Part model, mm, in its own coordinate system. A direction names the side the tool comes from. Coordinates: 2 decimals unless noted, no trailing zeros. Loops run counter-clockwise (first coordinate to the right, second up) from the corner with the lowest first, then second, coordinate; pieces in that order, holes last. Notation, with made-up numbers: M 22,-11.5 L 71,-11.5 A30 cw 71,25.5 Z; hole C 61,27 d5. An arc over 180 degrees is marked long. Use a Markdown table: item, result. Add a question column.
1) Band-saw the part on B-B (x = 24). List the corners of the cut face in (y, z).
2) Tool access for faces 4 (the flat face through (32, 3, -2)), 5 (the flat face through (24.79, -36.94, -1.14)), 6 (the cylindrical face through (8.22, 2.17, -1.14)): list every direction of +Z, -Z, +X, -X, +Y, -Y with a clear straight run to the whole face (end or side of a thin tool).
3) Wall check: probe 1 along Y at (x, z) = (26, -1.4); probe 2 along Y at (x, z) = (12, -1.75); probe 3 along Y at (x, z) = (25, -0.05). Give the ranges that are in metal, low to high. Write a range as from..to.
4) Band-saw the part on A-A (z = -1.6). List the corners of the cut face in (x, y), plus the area to 3 significant figures.
5) Band-saw the part on C-C (y = -20). List the corners of the cut face in (x, z), plus the area to 3 significant figures.
6) Band-saw the part on D-D (x = 12.25). List the corners of the cut face in (y, z).
7) Pin check, flat tips, straight feed: pin 1 Ø3.5 at (x, y) = (34.641, -20) entering from +Z; pin 2 Ø5.5 at (x, y) = (21.5, 37) entering from -Z; pin 3 Ø1 at (x, z) = (28.5, -1.5) entering from +Y. Stop position of each tip, or through.
8) Pull direction Y, two halves, no side cores. Call faces 1 (the cylindrical face through (8.202, -2.23, -1.138)), 2 (the flat face through (24.79, 36.94, -1.14)), 3 (the flat face through (28, 0, 0)): released by +Y, released by -Y, zero draft, split by the parting line, or undercut.
Autodesk Inventor part; units mm, degrees
ref_plane "YZ Plane" through (0, 0, 0) normal (1, 0, 0) x (0, 1, 0)
ref_plane "XZ Plane" through (0, 0, 0) normal (0, 1, 0) x (-1, 0, 0)
ref_plane "XY Plane" through (0, 0, 0) normal (0, 0, 1) x (1, 0, 0)
sketch "Sketch1" plane through (0, 0, 0) normal (0, 0, 1) x (1, 0, 0)
  circle A0 centre (0, 0) radius 7.5
  line L0 (-21.2869, 0) -> (22.3896, 0) construction
  line L1 (0, 21.9302) -> (0, -69.0741) construction
  line L2 (24.9778, -67) -> (-24.9778, -67) construction
  line L3 (-17.5, -57) -> (17.5, -57)
  line L4 (17.5, -57) -> (17.5, -67)
  line L5 (17.5, -67) -> (-17.5, -67)
  line L6 (-17.5, -67) -> (-17.5, -57)
  line L7 (-37.5278, -67) -> (-18.5, -67)
  line L8 (-18.5, -67) -> (-18.5, -56)
  line L9 (-17.5, -62) -> (17.5, -62) construction
  line L10 (-18.5, -59) -> (-22.5, -59)
  line L11 (-22.5, -59) -> (-22.5, -65)
  line L12 (-22.5, -65) -> (-18.5, -65)
  line L13 (-18.5, -65) -> (-18.5, -59)
  line L14 (-17.5, -60) -> (-21.5, -60)
  line L15 (-21.5, -60) -> (-21.5, -64)
  line L16 (-21.5, -64) -> (-17.5, -64)
  line L17 (-17.5, -64) -> (-17.5, -60)
  line L18 (-18.5, -56) -> (-28.8675, -56)
  line L19 (17.5, -60) -> (21.5, -60)
  line L20 (21.5, -60) -> (21.5, -64)
  line L21 (21.5, -64) -> (17.5, -64)
  line L22 (17.5, -64) -> (17.5, -60)
  line L23 (18.5, -67) -> (18.5, -56)
  line L24 (18.5, -67) -> (37.5278, -67)
  line L25 (18.5, -65) -> (22.5, -65)
  line L26 (22.5, -65) -> (22.5, -59)
  line L27 (22.5, -59) -> (18.5, -59)
  line L28 (18.5, -59) -> (18.5, -65)
  line L29 (18.5, -56) -> (28.8675, -56)
  line L30 (-23.7704, -40) -> (28.6931, -40) construction
  line L31 (-17.1762, -35.75) -> (17.1762, -35.75)
  line L32 (-22.0836, -44.25) -> (22.0836, -44.25)
  circle A1 centre (0, -40) radius 2.25
  line L33 (-7.5, -16) -> (7.5, -16)
  line L34 (7.5, -16) -> (7.5, -21)
  line L35 (7.5, -26) -> (-7.5, -26)
  line L36 (-7.5, -26) -> (-7.5, -24)
  line L37 (7.5, -21) -> (-7.5, -21) construction
  line L38 (-7.5, -18) -> (-3.5, -18)
  line L39 (-3.5, -18) -> (-3.5, -21)
  line L40 (-3.5, -24) -> (-7.5, -24)
  line L41 (-7.5, -24) -> (-7.5, -23)
  line L42 (-8.5, -19) -> (-4.5, -19)
  line L43 (-4.5, -19) -> (-4.5, -23)
  line L44 (-4.5, -23) -> (-8.5, -23)
  line L45 (-8.5, -23) -> (-8.5, -19)
  line L46 (7.5, -18) -> (3.5, -18)
  line L47 (3.5, -18) -> (3.5, -21)
  line L48 (3.5, -24) -> (7.5, -24)
  line L49 (7.5, -24) -> (7.5, -18)
  line L50 (8.5, -19) -> (4.5, -19)
  line L51 (4.5, -19) -> (4.5, -23)
  line L52 (4.5, -23) -> (8.5, -23)
  line L53 (8.5, -23) -> (8.5, -19)
  line L54 (-9.815, -19) -> (-31.1769, -56)
  line L55 (-7.5056, -19) -> (-28.8675, -56)
  line L56 (7.5056, -19) -> (28.8675, -56)
  line L57 (-4.5, -21) -> (-8.5, -21)
  line L58 (4.5, -21) -> (8.5, -21)
  line L59 (-21.5, -62) -> (-17.5, -62)
  line L60 (17.5, -62) -> (21.5, -62)
  line L61 (-22.5, -62) -> (-18.5, -62)
  line L62 (22.5, -62) -> (18.5, -62)
  line L63 (-7.5, -21) -> (-3.5, -21)
  line L64 (3.5, -21) -> (7.5, -21)
  line L65 (-28.8675, -56) -> (-31.1769, -56)
  line L66 (28.8675, -56) -> (31.1769, -56)
  line L67 (-10.8853, -24.8539) -> (-12.6173, -23.8539)
  line L68 (10.8875, -24.8576) -> (12.6195, -23.8576)
  line L69 (7.5, -23) -> (7.5, -24)
  line L70 (-7.5, -23) -> (-7.5, -21)
  line L71 (-7.5, -24) -> (-7.5, -16)
  line L72 (7.5, -24) -> (7.5, -26)
  line L73 (-7.5, -21) -> (-7.5, -18)
  line L74 (-3.5, -21) -> (-3.5, -24)
  line L75 (3.5, -21) -> (3.5, -24)
  line L76 (7.5, -21) -> (7.5, -23)
  line L77 (-18.4752, 0) -> (-9.2376, 16)
  line L78 (-9.2376, 16) -> (9.2376, 16)
  line L79 (9.2376, 16) -> (18.4752, 0)
  line L80 (18.4752, 0) -> (9.2376, -16)
  line L81 (9.2376, -16) -> (-9.2376, -16)
  line L82 (-9.2376, -16) -> (-18.4752, 0)
  line L83 (-77.3649, 0) -> (-38.6825, 67) construction
  line L84 (-38.6825, 67) -> (38.6825, 67) construction
  line L85 (38.6825, 67) -> (77.3649, 0) construction
  line L86 (77.3649, 0) -> (38.6825, -67) construction
  line L87 (38.6825, -67) -> (-38.6825, -67) construction
  line L88 (-38.6825, -67) -> (-77.3649, 0) construction
  line L89 (-9.2376, -16) -> (-38.6825, -67) construction
  line L90 (9.2376, -16) -> (38.6825, -67) construction
  line L91 (0, -16.7974) -> (0, -26) construction
  line L92 (9.815, -19) -> (31.1769, -56)
  line L93 (-8.5, -19) -> (-9.815, -19)
  line L94 (8.5, -19) -> (9.815, -19)
  line L95 (-8.5, -23) -> (-9.815, -23)
  line L96 (8.5, -23) -> (9.815, -23)
  line L97 (-31.1769, -56) -> (-37.5278, -67)
  line L98 (31.1769, -56) -> (37.5278, -67)
  circle A2 centre (12.25, 0) radius 2.25
  circle A3 centre (6.125, 10.6088) radius 2.25
  circle A4 centre (-6.125, 10.6088) radius 2.25
  circle A5 centre (-12.25, 0) radius 2.25
  circle A6 centre (-6.125, -10.6088) radius 2.25
  circle A7 centre (6.125, -10.6088) radius 2.25
  line L99 (22.3723, -32.75) -> (39.5485, -3)
  line L100 (27.2798, -41.25) -> (49.3634, -3)
  circle A8 centre (34.641, -20) radius 2.25
  line L101 (39.5485, 3) -> (22.3723, 32.75)
  line L102 (49.3634, 3) -> (27.2798, 41.25)
  circle A9 centre (34.641, 20) radius 2.25
  line L103 (17.1762, 35.75) -> (-17.1762, 35.75)
  line L104 (22.0836, 44.25) -> (-22.0836, 44.25)
  circle A10 centre (0, 40) radius 2.25
  line L105 (-22.3723, 32.75) -> (-39.5485, 3)
  line L106 (-27.2798, 41.25) -> (-49.3634, 3)
  circle A11 centre (-34.641, 20) radius 2.25
  line L107 (-39.5485, -3) -> (-22.3723, -32.75)
  line L108 (-49.3634, -3) -> (-27.2798, -41.25)
  circle A12 centre (-34.641, -20) radius 2.25
  line L109 (22.3723, -32.75) -> (27.2798, -41.25)
  line L110 (49.3634, -3) -> (51.0955, 0)
  line L111 (49.3634, 3) -> (51.0955, 0)
  line L112 (39.5485, -3) -> (41.2805, 0)
  line L113 (39.5485, 3) -> (41.2805, 0)
  line L114 (7.3612, 4.25) -> (38.8268, 4.25)
  line L115 (7.3612, -4.25) -> (38.8268, -4.25)
  arc A13 (8.5, 0) -> (7.3612, 4.25) centre (0, 0) ccw
  arc A14 (7.3612, -4.25) -> (8.5, 0) centre (0, 0) ccw
  arc A15 (7.3612, 4.25) -> (7.3612, -4.25) centre (0, 0) ccw
  line L116 (22.3723, 32.75) -> (27.2798, 41.25)
  circle A16 centre (26.0626, 35.75) radius 9.2862
  circle A17 centre (26.0626, -36.2861) radius 9.6381
  circle A18 centre (9.1575, 0.2994) radius 7.4055
  point P0 (0, -57)
  point P1 (0, -67)
  point P2 (0, -62)
  point P3 (0, -21)
  dimension "d0" = 15
  dimension "d16" = 10
  dimension "d20" = 6
  dimension "d21" = 4
  dimension "d22" = 4
  dimension "d23" = 1
  dimension "d24" = 1
  dimension "d25" = 35
  dimension "d27" = 3
  dimension "d28" = 4
  dimension "d29" = 1
  dimension "d30" = 6
  dimension "d31" = 4
  dimension "d32" = 1
  dimension "d34" = 3
  dimension "d35" = 27
  dimension "d39" = 4.5
  dimension "d41" = 2
  dimension "d42" = 2
  dimension "d44" = 10
  dimension "d45" = 4
  dimension "d46" = 6
  dimension "d48" = 4
  dimension "d49" = 1
  dimension "d50" = 4
  dimension "d52" = 6
  dimension "d53" = 4
  dimension "d54" = 4
  dimension "d55" = 1
  dimension "d56" = 4
  dimension "d57" = 15
  dimension "d60" = 2
  dimension "d81" = 16
  dimension "d83" = 67
  dimension "d84" = 1
  dimension "d86" = 2
  dimension "d87" = 1
  dimension "d88" = 5
  dimension "d89" = 3
  dimension "d90" = 3
  dimension "d112" = 4.5
  dimension "d113" = 2.5
  dimension "d116" = 360
  dimension "d120" = 360
  dimension "d122" = 2
  dimension "d123" = 2
  dimension "d124" = 1
extrude "Extrusion8" add sketch "Sketch1" against normal blind 2 contours L114 A18 L115 A14 A13 | L114 L79 L80 L115 A18 | L114 L101 L113 L112 L99 L115 L80 L79 | L101 A16 L102 L111 L110 L100 A17 L99 L112 L113 | L101 L116 L102 A16 | A17 L100 L109 L99 picked at (27.7483, 34.7719)
extrude "Extrusion9" add sketch "Sketch1" against normal blind 0.3 contours A0 A18 | A0 A18 A15 A13 A14 | A18 L114 A15 | A15 L115 A18 | L114 A18 L115 A14 A13 | A16 L102 L116 L101 | L101 L116 L102 A16 | A17 L100 L109 L99 | L99 L109 L100 A17 L92 | L92 A17 L56 | L56 L31 A17 | A17 L32 L56 | L56 L32 A17 L31 picked at (5.5176, 0.5972)
equation "\"d20\" = hinge_w"
equation "\"d21\" = hinge_d"
equation "\"d22\" = hinge_w - 2 * hinge_sp"
equation "\"d23\" = hinge_sp"
equation "\"d24\" = sp"
equation "\"d28\" = hinge_w - 2 * hinge_sp"
equation "\"d29\" = sp"
equation "\"d30\" = hinge_w"
equation "\"d31\" = hinge_d"
equation "\"d32\" = hinge_sp"
equation "\"d39\" = screw"
equation "\"d45\" = hinge_d"
equation "\"d46\" = hinge_w"
equation "\"d48\" = hinge_d"
equation "\"d49\" = hinge_sp"
equation "\"d50\" = hinge_w - 2 * hinge_sp"
equation "\"screw\" = 4.5"
equation "\"k\" = 0.4"
equation "\"sp\" = 1"
equation "\"d14\" = sp"
equation "\"d15\" = sp"
equation "\"d19\" = sp"
equation "\"hinge_d\" = 4"
equation "\"hinge_w\" = 6"
equation "\"hinge_sp\" = 1"
properties part number "RobotBase" material "Glass"
Entries:
| question | item | result |
|---|---|---|
| 1 | outline | M -45.7,-0.3 L -35.57,-0.3 L -35.57,-2 L -29.93,-2 L -29.93,-0.3 L -26.87,-0.3 L -26.87,0 L -45.7,0 Z; M -4.25,-2 L 4.25,-2 L 4.25,0 L -4.25,0 Z; M 26.7,-0.3 L 29.93,-0.3 L 29.93,-2 L 35.57,-2 L 35.57,-0.3 L 44.8,-0.3 L 44.8,0 L 26.7,0 Z |
| 2 | face 4 | -Z, +X, -X, +Y, -Y |
| 2 | face 5 | -Z, -X, -Y |
| 2 | face 6 | -Z, -X |
| 3 | probe 1 | -39.03..-26.47, -4.25..4.25, 26.47..39.03 |
| 3 | probe 2 | -4.25..-2.24, 2.24..4.25 |
| 3 | probe 3 | -45.87..-26.71, -4.25..4.25, 26.52..44.98 |
| 4 | outline | M 7.36,-4.25 L 38.83,-4.25 L 22.37,-32.75 L 27.28,-41.25 L 49.36,-3 L 51.1,0 L 49.36,3 L 27.28,41.25 L 22.37,32.75 L 38.83,4.25 L 7.36,4.25 A8.5 cw 8.5,0 A8.5 cw Z; hole C 12.25,0 d4.5; hole C 34.64,-20 d4.5; hole C 34.64,20 d4.5 |
| 4 | area | 950 mm2 |
| 5 | outline | M 29.73,-2 L 32.39,-2 L 32.39,0 L 29.73,0 Z; M 36.89,-2 L 39.55,-2 L 39.55,0 L 36.89,0 Z |
| 5 | area | 10.6 mm2 |
| 6 | outline | M -6.43,-0.3 L -4.25,-0.3 L -4.25,-2 L -2.25,-2 L -2.25,0 L -6.43,0 Z; M 2.25,-2 L 4.25,-2 L 4.25,-0.3 L 7.03,-0.3 L 7.03,0 L 2.25,0 Z |
| 7 | pin 1 | through |
| 7 | pin 2 | z = -0.3 |
| 7 | pin 3 | y = 40 |
| 8 | face 1 | undercut |
| 8 | face 2 | released by +Y |
| 8 | face 3 | zero draft |
